Check sheet for the modelled part. Datum: model origin and axes. Units: mm. A direction names the side the tool comes from. Coordinates: 2 decimals unless noted, no trailing zeros. Order: outer loops, then holes, each group sorted by start corner. A loop starts at its lowest first (then second) coordinate and runs counter-clockwise, first axis right, second up.
from build123d import *

# Parameters (mm, degrees)
SKETCH1_W                                        = 50
SKETCH1_H                                        = 40
BOSS_EXTRUDE1_DEPTH                              = 4
SKETCH2_W                                        = 7.705962758
SKETCH2_H                                        = 14.539090136
CUT_EXTRUDE1_DEPTH                               = 122.811546491
SKETCH3_W                                        = 10.372123492
SKETCH3_H                                        = 14.267331442
CUT_EXTRUDE2_DEPTH                               = 122.811546491
CBORE_FOR_M2_PAN_HEAD_MACHINE_SCREW1_D           = 2.4
CBORE_FOR_M2_PAN_HEAD_MACHINE_SCREW1_CBORE_D     = 5
CBORE_FOR_M2_PAN_HEAD_MACHINE_SCREW1_CBORE_DEPTH = 1.6
SKETCH6_W                                        = 47
SKETCH6_H                                        = 37
BOSS_EXTRUDE2_DEPTH                              = 4
SKETCH7_R                                        = 4
BOSS_EXTRUDE3_DEPTH                              = 5
F_2_7_2_7_DIAMETER_HOLE1_D                       = 2.7
F_2_7_2_7_DIAMETER_HOLE1_DEPTH                   = 4
F_2_7_2_7_DIAMETER_HOLE1_TIP                     = 0.811161836
CUT_EXTRUDE3_DEPTH                               = 6.5


with BuildPart() as part:
    # Sketch1 → Boss-Extrude1 (new body)
    with BuildSketch(Plane(origin=(0, 0, 34.811611197), x_dir=(-1, 0, 0), z_dir=(0, 0, -1))):
        with Locations((1.46446617, 98.834695645)):
            Rectangle(SKETCH1_W, SKETCH1_H)
    extrude(amount=-BOSS_EXTRUDE1_DEPTH)

    # Sketch2 → Cut-Extrude1 (cut, through all)
    with BuildSketch(Plane.XY.offset(38.811611197)):
        with Locations((19.682552451, 98.267628733)):
            Rectangle(SKETCH2_W, SKETCH2_H)
    extrude(amount=-CUT_EXTRUDE1_DEPTH, mode=Mode.SUBTRACT)

    # Sketch3 → Cut-Extrude2 (cut, through all)
    with BuildSketch(Plane.XY.offset(38.811611197)):
        with Locations((1.539593072, 98.131749386)):
            Rectangle(SKETCH3_W, SKETCH3_H)
    extrude(amount=-CUT_EXTRUDE2_DEPTH, mode=Mode.SUBTRACT)

    # CBORE for M2 Pan Head Machine Screw1 (through all)
    with Locations(Plane(origin=(0, 0, 34.811611197), x_dir=(-1, 0, 0), z_dir=(0, 0, -1))):
        with Locations((-3.156646479, 84.016340669), (-19.156646479, 84.016340669), (-19.156646479, 114.016340669), (-3.156646479, 114.016340669)):
            CounterBoreHole(CBORE_FOR_M2_PAN_HEAD_MACHINE_SCREW1_D / 2, CBORE_FOR_M2_PAN_HEAD_MACHINE_SCREW1_CBORE_D / 2, CBORE_FOR_M2_PAN_HEAD_MACHINE_SCREW1_CBORE_DEPTH)

    # Sketch6 → Boss-Extrude2 (add)
    with BuildSketch(Plane.XY.offset(38.811611197)):
        with Locations((-49.96446617, 97.334695645)):
            Rectangle(SKETCH6_W, SKETCH6_H)
    extrude(amount=-BOSS_EXTRUDE2_DEPTH)

    # Sketch7 → Boss-Extrude3 (add)
    with BuildSketch(Plane.XY.offset(38.811611197)):
        with Locations(Location((-68.96446617, 111.334695645, 0), (0, 0, 180))):
            Circle(SKETCH7_R)
        with Locations(Location((-31.96446617, 111.334695645, 0), (0, 0, 180))):
            Circle(SKETCH7_R)
        with Locations(Location((-68.96446617, 83.334695645, 0), (0, 0, 180))):
            Circle(SKETCH7_R)
        with Locations(Location((-31.96446617, 83.334695645, 0), (0, 0, 180))):
            Circle(SKETCH7_R)
    extrude(amount=BOSS_EXTRUDE3_DEPTH)

    # Ø2.7 (2.7) Diameter Hole1
    with Locations(Plane.XY.offset(43.811611197)):
        with Locations((-68.96446617, 111.334695645), (-31.96446617, 111.334695645), (-31.96446617, 83.334695645), (-68.96446617, 83.334695645)):
            Hole(F_2_7_2_7_DIAMETER_HOLE1_D / 2, depth=F_2_7_2_7_DIAMETER_HOLE1_DEPTH)
            with Locations((0, 0, -(F_2_7_2_7_DIAMETER_HOLE1_DEPTH + F_2_7_2_7_DIAMETER_HOLE1_TIP / 2))):  # 118° drill point
                Cone(0, F_2_7_2_7_DIAMETER_HOLE1_D / 2, F_2_7_2_7_DIAMETER_HOLE1_TIP, mode=Mode.SUBTRACT)

    # Sketch10 → Cut-Extrude3 (cut)
    with BuildSketch(Plane.XY.offset(43.811611197)):
        Polygon((-67.521090497, 113.834695645), (-70.407841843, 113.834695645), (-71.851217516, 111.334695645), (-70.407841843, 108.834695645), (-67.521090497, 108.834695645), (-66.077714824, 111.334695645), align=None)
        Polygon((-67.521090497, 85.834695645), (-70.407841843, 85.834695645), (-71.851217516, 83.334695645), (-70.407841843, 80.834695645), (-67.521090497, 80.834695645), (-66.077714824, 83.334695645), align=None)
        Polygon((-30.521090497, 113.834695645), (-33.407841843, 113.834695645), (-34.851217516, 111.334695645), (-33.407841843, 108.834695645), (-30.521090497, 108.834695645), (-29.077714824, 111.334695645), align=None)
        Polygon((-30.521090497, 85.834695645), (-33.407841843, 85.834695645), (-34.851217516, 83.334695645), (-33.407841843, 80.834695645), (-30.521090497, 80.834695645), (-29.077714824, 83.334695645), align=None)
    extrude(amount=-CUT_EXTRUDE3_DEPTH, mode=Mode.SUBTRACT)


solid = part.part
(1) Cross-section at A-A (z = 41.25). Enter the section's corners in (x, y).
Filled in:
outline: circle Ø8 at (-68.96, 83.33); circle Ø8 at (-68.96, 111.33); circle Ø8 at (-31.96, 83.33); circle Ø8 at (-31.96, 111.33); hole (-71.85, 83.33) - (-70.41, 80.83) - (-67.52, 80.83) - (-66.08, 83.33) - (-67.52, 85.83) - (-70.41, 85.83) - close; hole (-71.85, 111.33) - (-70.41, 108.83) - (-67.52, 108.83) - (-66.08, 111.33) - (-67.52, 113.83) - (-70.41, 113.83) - close; hole (-34.85, 83.33) - (-33.41, 80.83) - (-30.52, 80.83) - (-29.08, 83.33) - (-30.52, 85.83) - (-33.41, 85.83) - close; hole (-34.85, 111.33) - (-33.41, 108.83) - (-30.52, 108.83) - (-29.08, 111.33) - (-30.52, 113.83) - (-33.41, 113.83) - close
(2) Thickness scan on probe 1 along Y at (x, z) = (3, 38); probe 2 along X at (y, z) = (82.5, 40.75); probe 3 along X at (y, z) = (113, 37.5). Record the ranges inside material, lowest first.
Filled in:
probe 1: y = 78.83 to 82.83, 85.21 to 91, 105.27 to 112.83, 115.21 to 118.83
probe 2: x = -72.88 to -71.37, -66.56 to -65.05, -35.88 to -34.37, -29.56 to -28.05
probe 3: x = -73.46 to -70.89, -67.04 to -33.89, -30.04 to 2.52, 3.79 to 18.52, 19.79 to 23.54
(3) Cross-section at B-B (y = 95.5). Enter the section's corners in (x, z).
Filled in:
outline: (-73.46, 34.81) - (-3.65, 34.81) - (-3.65, 38.81) - (-73.46, 38.81) - close; (6.73, 34.81) - (15.83, 34.81) - (15.83, 38.81) - (6.73, 38.81) - close
(4) Cross-section at D-D (y = 88.5). Enter the section's corners in (x, z).
Filled in:
outline: (-73.46, 34.81) - (23.54, 34.81) - (23.54, 38.81) - (-73.46, 38.81) - close
(5) Tool access check on faces 5 (the flat face through (6.726, 98, 37)), 6 (the flat face through (-50, 115.835, 37)), 7 (the flat face through (2, 115, 36.412)), 8 (the cylindrical face through (-68.44, 107.37, 41.28)). Record the directions out of +Z, -Z, +X, -X, +Y, -Y that give a thin tool (end or side, any length) a straight path to the whole face; none if there is none.
Filled in:
face 5: +Z, -Z
face 6: +Z, -Z, -X, +Y
face 7: -Z
face 8: +Z
(6) Cross-section at C-C (x = -19). Enter the section's corners in (y, z).
Filled in:
outline: (78.83, 34.81) - (118.83, 34.81) - (118.83, 38.81) - (78.83, 38.81) - close
(7) Release check for a two-part mould opening along Y. For faces 1 (the flat face through (20, 105.537, 37)), 2 (the flat face through (-69, 86, 43.812)), 3 (the flat face through (-1, 118.835, 37)), 4 (the cylindrical face through (2.897, 82.845, 37.628)) record: +Y half, -Y half, draft (parallel to the pull), parting line (faces both ways), or undercut.
Filled in:
face 1: undercut
face 2: draft
face 3: +Y half
face 4: undercut
(8) Go/stop test with flat-tipped pins: P1, Ø1.5, axis at x = 20, y = 115, coming from the -Z side; P2, Ø4, axis at x = -39.5, z = 39.5, coming from the +Y side; P3, Ø1, axis at x = 8, y = 112.5, coming from the +Z side. Record where each tip stops, or that it passes through.
Filled in:
P1: stops at z = 36.41
P2: stops at y = 115.83
P3: stops at z = 38.81
